Autodesk Inventor part; units mm, degrees
ref_plane "Arbeitsebene1" through (0, 0, 0) normal (0, 1, 0) x (-1, 0, 0)
ref_plane "YZ Plane" through (0, 0, 0) normal (1, 0, 0) x (0, 1, 0)
ref_plane "XY Plane" through (0, 0, 0) normal (0, 0, 1) x (1, 0, 0)
sketch "Skizze4" plane through (0, 0, 0) normal (0, 0, 1) x (1, 0, 0)
  line L0 (0, 0) -> (0, 7)
  line L1 (0, 7) -> (11.5, 7)
  line L2 (11.5, 7) -> (12, 6.134)
  line L3 (12, 6.134) -> (12.5, 7)
  line L4 (12.5, 7) -> (16.5, 7)
  line L5 (16.5, 7) -> (17, 6.134)
  line L6 (17, 6.134) -> (17.5, 7)
  line L7 (17.5, 7) -> (21.5, 7)
  line L8 (21.5, 7) -> (22, 6.134)
  line L9 (22, 6.134) -> (22.5, 7)
  line L10 (22.5, 7) -> (26.1132, 7)
  line L11 (26.1132, 7) -> (29, 2)
  line L12 (29, 2) -> (29, 0)
  line L13 (29, 0) -> (0, 0)
  line L14 (12, 6.134) -> (12, 7.9514) construction
  line L15 (17, 6.134) -> (17, 8.1262) construction
  line L16 (22, 6.134) -> (22, 7.8166) construction
  point P0 (29, 1)
  dimension "d7" = 1
  dimension "d8" = 60
  dimension "d9" = 4
  dimension "d10" = 14
  dimension "d11" = 7
  dimension "d12" = 29
  dimension "d13" = 12
  dimension "d14" = 17
  dimension "d15" = 30
  dimension "d16" = 1
revolve "Umdrehung1" add sketch "Skizze4" angle 360 about axis through (29, 0, 0) along (-1, 0, 0)
sketch "Skizze5" plane through (0, 0, 0) normal (-1, 0, 0) x (0, 0, 1)
  circle A0 centre (0, 0) radius 7
  line L0 (-7, 0.6) -> (7, 0.6)
  line L1 (7, 0.6) -> (7, -0.6)
  line L2 (7, -0.6) -> (-7, -0.6)
  line L3 (-7, -0.6) -> (-7, 0.6)
  circle A1 centre (0, 0) radius 7
  line L4 (-7, 0) -> (7.2864, 0) construction
  dimension "d18" = 1.2
extrude "Extrusion1" cut sketch "Skizze5" against normal blind 8 contours A0 L2 L0 | L1 L2 A0 | A0 L0 L1 | A0 L3 L0 | L2 L3 A0
ref_plane "Arbeitsebene1" through (0, 0, 0) normal (0, 1, 0) x (-1, 0, 0)
sketch "Skizze6" plane through (0, 0, 0) normal (0, 1, 0) x (-1, 0, 0)
  point P0 (0, 0)
  point P1 (-4, 0)
  dimension "d22" = 4
hole "Bohrung1" at (4, 0, 0) direction (0, -1, 0) diameter 2 end through all both
properties part number "arbeitskolben" material "Blei"
Input: part model. Units: mm. Frame: model coordinates. A direction names the side the tool comes from. Coordinates: 2 decimals unless noted, no trailing zeros. Loops run counter-clockwise (first coordinate to the right, second up) from the corner with the lowest first, then second, coordinate; pieces in that order, holes last.
Q1. Cut plane B-B (z = 0). Give the number of separate pieces and of enclosed holes in the cut face, then the cut area to 3 significant figures.
Q2. Draft query along Y for faces 3 (the face through (8, 0, 0)), 4 (the face through (3, 4, 0)), 5 (the face through (5.83, 6.466, -2.681)). Return one class per face: +Y half, -Y half, draft (parallel to the pull), parting line (faces both ways), or undercut.
Q3. Material intervals for line 1 (Y direction, x = 7.75, z = -0.25); line 2 (Y direction, x = 2.5, z = 2.5); line 3 (X direction, y = 4.75, z = 0), sorted ascending.
Q4. Cut plane A-A (x = 4). Output: boundary loops of the cut face in (y, z).
Q5. Set-up query: faces 1 (the face through (4, 0.6, -2)), 2 (the face through (3, -4, 0)). Return all of +Z, -Z, +X, -X, +Y, -Y with unobstructed straight access to the full face (end or side cutting, diameter ignored); none if empty.
Q6. Contact query for flat-ended pins moving along their axis: pin 1 (0.6 mm diameter, centred on y = 0, z = -1.5, fed in from -X); pin 2 (1 mm diameter, centred on y = -4.5, z = 0.5, fed in from +X); pin 3 (2 mm diameter, centred on x = 24, y = 5, fed in from +Z); pin 4 (1.6 mm diameter, centred on x = 4, z = 0, fed in from -Y). Output: stop coordinate, or through.
Q7. Cut plane C-C (x = 8.5). Output: boundary loops of the cut face in (y, z).
Working result:
1. separate pieces: 3
1. enclosed holes: 0
1. area: 354 mm2
2. face 3: undercut
2. face 4: draft
2. face 5: parting line
3. line 1: y = -7 to -0.6, 0.6 to 7
3. line 2: y = -6.54 to -0.6, 0.6 to 6.54
3. line 3: x = 0 to 3, 5 to 27.41
4. outline: (-6.93, -1) arc R7 ccw to (-0.6, -6.97) - (-0.6, -1) - close; (-6.93, 1) - (-0.6, 1) - (-0.6, 6.97) arc R7 ccw to start; (0.6, -6.97) arc R7 ccw to (6.93, -1) - (0.6, -1) - close; (0.6, 1) - (6.93, 1) arc R7 ccw to (0.6, 6.97) - close
5. face 1: +Z, -Z, -X
5. face 2: +Y, -Y
6. pin 1: stops at x = 8
6. pin 2: stops at x = 27.83
6. pin 3: stops at z = 5.74
6. pin 4: passes through
7. outline: circle Ø14 at (0, 0)
